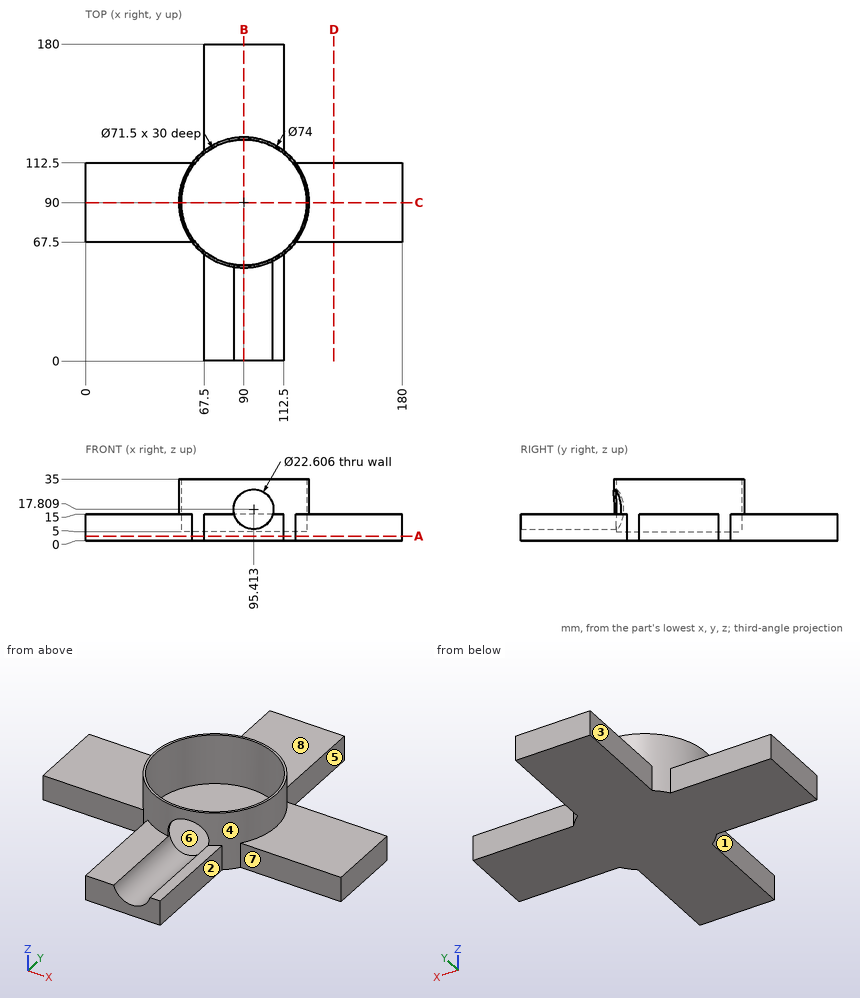
The drawing under review shows one solid part. Ordinate dimensions are in mm from its lowest x, y, z. A direction names the side the tool comes from. Coordinates: 2 decimals unless noted, no trailing zeros. Write each loop counter-clockwise with the first axis right and the second up, starting at its lowest first coordinate (ties: lowest second). Pieces come first, ordered by that corner, then holes. Notation, with made-up numbers: (35.5, -8.75) -> (59.5, -8.75) arc R31 ccw to (59.5, 21.25) -> close; hole circle Ø2 at (-16.5, 78.25). An arc over 180 degrees is marked (long way). Write each question's results on one line, items separated by ' | '. Start each with the question number.
1) For the marked faces 1, 2, 3, 4 and 5, list the 3-axis set-ups (+Z, -Z, +X, -X, +Y, -Y) from which the entire face can be reached by the end or side of a thin tool; tool diameter is ignored.
2) Consider section B-B (x = 90). Write out the cut boundary in (y, z).
3) Consider section A-A (z = 2.5). Write out the cut boundary in (x, y), plus the area to 3 significant figures.
4) Consider section C-C (y = 90). Write out the cut boundary in (x, z).
5) Consider section D-D (x = 141). Write out the cut boundary in (y, z), plus the area to 3 significant figures.
6) Wall thickness on L1, parallel to Z at x = 135.5, y = 79; L2, parallel to Y at x = 90, z = 29.5; L3, parallel to Y at x = 167, z = 3.5: over which ranges is each line inside the solid? List them lowest first. Write a range as [from, to].
7) The part is to be moulded in two halves that separate along Y. For the marked faces 6, 7 and 8, say which applies: +Y half, -Y half, draft (parallel to the pull), parting line (faces both ways), or undercut.
8) Insertion check: pin 1 (4.5 mm diameter, centred on y = 34.5, z = 5.5, fed in from -X); pin 2 (7.5 mm diameter, centred on x = 45, z = 5, fed in from -Y); pin 3 (3 mm diameter, centred on x = 89, z = 18, fed in from -Y). Each pin has a flat end and moves straight along its axis. Give the tip position at first contact, or say it passes through.
Geometry says:
1) face 1: +Z, -Z, -X, -Y | face 2: +Z, -Z, +X, -Y | face 3: +Z, -Z, -X, +Y | face 4: +Z | face 5: +Z, -Z, +X, +Y
2) outline: (0, 0) -> (180, 0) -> (180, 15) -> (127, 15) -> (127, 35) -> (125.75, 35) -> (125.75, 5) -> (54.25, 5) -> (54.25, 7.89) -> (0, 7.89) -> close; (53, 27.73) -> (54.25, 27.73) -> (54.25, 35) -> (53, 35) -> close
3) outline: (0, 67.5) -> (60.63, 67.5) arc R37 ccw to (67.5, 60.63) -> (67.5, 0) -> (112.5, 0) -> (112.5, 60.63) arc R37 ccw to (119.37, 67.5) -> (180, 67.5) -> (180, 112.5) -> (119.37, 112.5) arc R37 ccw to (112.5, 119.37) -> (112.5, 180) -> (67.5, 180) -> (67.5, 119.37) arc R37 ccw to (60.63, 112.5) -> (0, 112.5) -> close | area: 14,300 mm^2
4) outline: (0, 0) -> (180, 0) -> (180, 15) -> (127, 15) -> (127, 35) -> (125.75, 35) -> (125.75, 5) -> (54.25, 5) -> (54.25, 35) -> (53, 35) -> (53, 15) -> (0, 15) -> close
5) outline: (67.5, 0) -> (112.5, 0) -> (112.5, 15) -> (67.5, 15) -> close | area: 675 mm^2
6) L1: [0, 15] | L2: [53, 54.25], [125.75, 127] | L3: [67.5, 112.5]
7) face 6: undercut | face 7: -Y half | face 8: draft
8) pin 1: x = 67.5 | pin 2: y = 67.5 | pin 3: y = 125.66
